```python
from build123d import *

# Parameters (mm, degrees)
SKETCH1_R           = 0.835
BOSS_EXTRUDE1_DEPTH = 20
CHAMFER1_SIZE       = 0.1


with BuildPart() as part:
    # Sketch1 → Boss-Extrude1 (new body)
    with BuildSketch(Plane(origin=(0, 0, 0), x_dir=(1, 0, 0), z_dir=(0, 1, 0))):
        with BuildLine():
            Line((2.776760362, 5.133225937), (0.142399779, 0.609778229))
            Line((0.142399779, 0.609778229), (0.0893221, 0.518638806))
            ThreePointArc((0.0893221, 0.518638806), (0.636251586, 0.056736494), (1.155841613, -0.435718389))
            Line((1.155841613, -0.435718389), (-7.720764547, -9.245763982))
            Line((-7.720764547, -9.245763982), (-4.441814223, 2.809787769))
            ThreePointArc((-4.441814223, 2.809787769), (-3.757359805, 2.60387674), (-3.085793629, 2.359180862))
            Line((-3.085793629, 2.359180862), (-3.030668296, 2.453836303))
            Line((-3.030668296, 2.453836303), (-0.394624771, 6.980173781))
            ThreePointArc((-0.394624771, 6.980173781), (2.114541718, 7.642392425), (2.776760362, 5.133225937))
        make_face()
        with Locations(Location((1.191067796, 6.056699859, 0), (0, 0, 270))):
            Circle(SKETCH1_R, mode=Mode.SUBTRACT)
    extrude(amount=BOSS_EXTRUDE1_DEPTH)

    # Chamfer1
    chamfer1_edges = [part.edges().sort_by_distance(p)[0] for p in [
        (-3.282461467, 20, 4.840741186),
        (-3.282461467, 0, 4.840741186),
        (-6.081289385, 20, 3.217988107),
        (-6.081289385, 0, 3.217988107),
    ]]
    chamfer(chamfer1_edges, length=CHAMFER1_SIZE)


solid = part.part
```
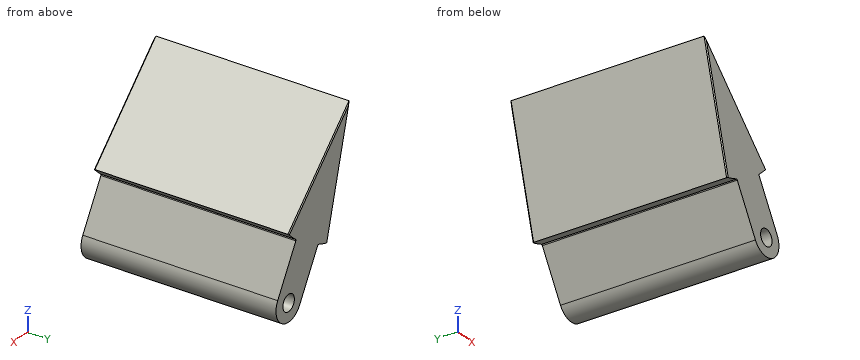
Geometry: final body of the model. Coordinates: model frame, mm. Round coordinates to 2 decimals unless told otherwise and drop trailing zeros. Write each loop counter-clockwise with the first axis right and the second up, starting at its lowest first coordinate (ties: lowest second). Pieces come first, ordered by that corner, then holes. Notation, with made-up numbers: (9, 75.25) -> (48, 75.25) arc R17 cw to (48, 91.25) -> close; hole circle Ø9 at (34, 29.25). An arc over 180 degrees is marked (long way). Use CSV: the item, a comma, the result in double quotes. Start each with the question number.
Q1. Section D-D (z = 3.5). Return loops of the section in (x, y), plus the area to 3 significant figures.
Q2. First-contact query: pin 1 Ø2 at (x, z) = (1.19, -6.06) entering from -Y; pin 2 Ø3 at (y, z) = (5, 6) entering from -X; pin 3 Ø2 at (x, y) = (-3, 6) entering from +Z; pin 4 Ø5 at (y, z) = (16.5, -5.5) entering from -X. Flat tips, straight axial feed; report the tip coordinate or a pass-through.
Q3. Section B-B (x = -4). Return loops of the section in (y, z), plus the area to 3 significant figures.
Q4. Section A-A (y = 6.75). Return loops of the section in (x, z) (3 decimals).
Q5. Line query: L1, parallel to Z at x = 0.75, y = 2.5; L2, parallel to X at y = 5, z = -6; L3, parallel to Z at x = 0.5, y = 2.75. Output: solid intervals per line, ascending.
Q6. Section C-C (z = 1.5). Return loops of the section in (x, y).
Result sheet:
1,outline,"(-6.16, 0.1) -> (-6.05, 0) -> (-2.07, 0) -> (-1.93, 0.1) -> (-1.93, 19.9) -> (-2.07, 20) -> (-6.05, 20) -> (-6.16, 19.9) -> close"
1,area,"84.5 mm²"
2,pin 1,"y = 0"
2,pin 2,"x = -7.25"
2,pin 3,"z = 5.55"
2,pin 4,"x = -2.71"
3,outline,"(0, -2.68) -> (20, -2.68) -> (20, 5.41) -> (19.9, 5.55) -> (0.1, 5.55) -> (0, 5.41) -> close"
3,area,"165 mm²"
4,outline,"(-7.721, 9.246) -> (-4.442, -2.81) arc R12.5 ccw to (-3.086, -2.359) -> (-0.395, -6.98) arc R1.835 ccw to (2.777, -5.133) -> (0.089, -0.519) arc R12.5 ccw to (1.156, 0.436) -> close; hole circle Ø1.67 at (1.191, -6.057)"
5,L1,"-7.84 to -6.77, -5.35 to -1.65, 0.05 to 0.84"
5,L2,"-0.97 to 0.36, 2.02 to 3.03"
5,L3,"-7.76 to -6.53, -5.59 to -1.22, -0.18 to 1.09"
6,outline,"(-5.61, 0.1) -> (-5.51, 0) -> (-0.06, 0) -> (0.08, 0.1) -> (0.08, 19.9) -> (-0.06, 20) -> (-5.51, 20) -> (-5.61, 19.9) -> close"
